For this review, take the finished solid that the model builds, in its own axes (mm). Face numbers are marked on the shaded views. A direction names the side the tool comes from. Coordinates: 2 decimals unless noted, no trailing zeros. Write each loop counter-clockwise with the first axis right and the second up, starting at its lowest first coordinate (ties: lowest second). Pieces come first, ordered by that corner, then holes.
1) We need section A-A on x = 45. Write out the cut boundary in (y, z), then the cut area to 3 significant figures.
2) Insertion check: P1, Ø14.5, axis at y = 45, z = 20, coming from the -X side; P2, Ø12, axis at x = 7, z = 26.5, coming from the +Y side; P3, Ø4, axis at x = 80, z = 10, coming from the -Y side; P4, Ø10, axis at y = 24, z = 14.5, coming from the -X side. Each pin has a flat end and moves straight along its axis. Give the tip position at first contact, or say it passes through.
3) We need section D-D on x = 21. Write out the cut boundary in (y, z).
4) To check wall thickness, follow line 1 along Z through (x, y) = (10, 10); line 2 along X through (y, z) = (7, 10); line 3 along Y through (x, z) = (11.5, 24). State the ranges of each line that lie inside material, in increasing order.
5) We need section C-C on z = 28. Give the number of separate pieces and of enclosed holes in the cut face, then the cut area to 3 significant figures.
6) We need section B-B on y = 24. Write out the cut boundary in (x, z).
7) For the marked faces 1, 2 and 3, list the 3-axis set-ups (+Z, -Z, +X, -X, +Y, -Y) from which the entire face can be reached by the end or side of a thin tool; tool diameter is ignored.
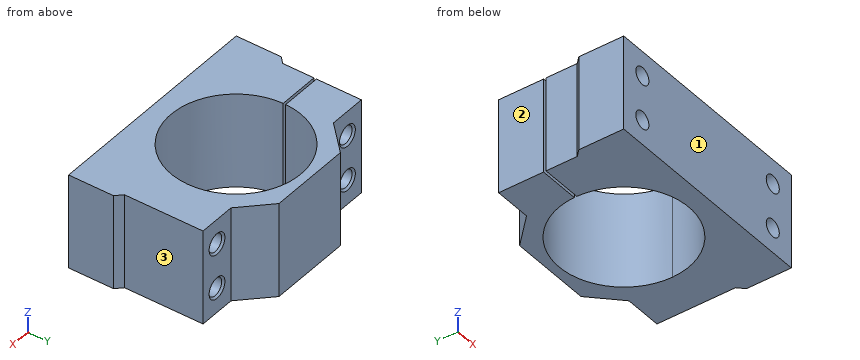
from build123d import *

# Parameters (mm, degrees)
AUFSATZ_LINEAR_AUSTRAGEN1_DEPTH          = 38
SKIZZE2_R                                = 26
SCHNITT_LINEAR_AUSTRAGEN1_DEPTH          = 38
SKIZZE3_W                                = 17
SKIZZE3_H                                = 1
SCHNITT_LINEAR_AUSTRAGEN2_DEPTH          = 38
F_7_0_7_DURCHMESSER_BOHRUNG4_D           = 7
F_7_0_7_DURCHMESSER_BOHRUNG4_CSINK_D     = 8.5
F_7_0_7_DURCHMESSER_BOHRUNG4_CSINK_ANGLE = 90


with BuildPart() as part:
    # Skizze1 → Aufsatz-Linear austragen1 (new body)
    with BuildSketch(Plane.XY):
        Polygon((0, 0), (0, 18), (2.5, 20.5), (2.5, 52), (17.5, 52), (28.51, 63.01), (61.49, 63.01), (72.5, 52), (87.5, 52), (87.5, 20.5), (90, 18), (90, 0), align=None)
    extrude(amount=AUFSATZ_LINEAR_AUSTRAGEN1_DEPTH)

    # Skizze2 → Schnitt-Linear austragen1 (cut)
    with BuildSketch(Plane.XY.offset(38)):
        with Locations((45, 33.5)):
            Circle(SKIZZE2_R)
    extrude(amount=-SCHNITT_LINEAR_AUSTRAGEN1_DEPTH, mode=Mode.SUBTRACT)

    # Skizze3 → Schnitt-Linear austragen2 (cut)
    with BuildSketch(Plane.XY.offset(38)):
        with Locations((11, 33.5)):
            Rectangle(SKIZZE3_W, SKIZZE3_H)
    extrude(amount=-SCHNITT_LINEAR_AUSTRAGEN2_DEPTH, mode=Mode.SUBTRACT)

    # Ø7.0 (7) Durchmesser Bohrung4 (through all)
    with Locations(Plane(origin=(0, 52, 0), x_dir=(1, 0, 0), z_dir=(0, 1, 0))):
        with Locations((10, -10), (10, -28), (80, -28), (80, -10)):
            CounterSinkHole(F_7_0_7_DURCHMESSER_BOHRUNG4_D / 2, F_7_0_7_DURCHMESSER_BOHRUNG4_CSINK_D / 2, counter_sink_angle=F_7_0_7_DURCHMESSER_BOHRUNG4_CSINK_ANGLE)


solid = part.part
Result:
1. outline: (0, 0) - (7.5, 0) - (7.5, 38) - (0, 38) - close; (59.5, 0) - (63.01, 0) - (63.01, 38) - (59.5, 38) - close
1. area: 418 mm2
2. P1: stops at x = 2.5
2. P2: stops at y = 52
2. P3: passes through
2. P4: stops at x = 1
3. outline: (0, 0) - (23.5, 0) - (23.5, 38) - (0, 38) - close; (43.5, 0) - (55.5, 0) - (55.5, 38) - (43.5, 38) - close
4. line 1: z = 0 to 6.5, 13.5 to 24.5, 31.5 to 38
4. line 2: x = 0 to 6.5, 13.5 to 76.5, 83.5 to 90
4. line 3: y = 0 to 33, 34 to 52
5. separate pieces: 4
5. enclosed holes: 0
5. area: 2,140 mm2
6. outline: (2.5, 0) - (20.8, 0) - (20.8, 38) - (2.5, 38) - close; (69.2, 0) - (87.5, 0) - (87.5, 38) - (69.2, 38) - close; hole circle Ø7 at (10, 10); hole circle Ø7 at (10, 28); hole circle Ø7 at (80, 10); hole circle Ø7 at (80, 28)
7. face 1: +Z, -Z, +X, -X, -Y
7. face 2: +Z, -Z, -X, +Y
7. face 3: +Z, -Z, +X, +Y
